Here's how the part is built. I have some questions about the finished solid (model axes, mm). A direction names the side the tool comes from. Round coordinates to 2 decimals unless told otherwise and drop trailing zeros. Write each loop counter-clockwise with the first axis right and the second up, starting at its lowest first coordinate (ties: lowest second). Pieces come first, ordered by that corner, then holes. Notation, with made-up numbers: (80, -29.75) - (121, -29.75) arc R21 ccw to (121, -12.75) - close; hole circle Ø10 at (42.25, 7). An arc over 180 degrees is marked (long way). Return JSON: item names as keys, results as strings. Group by question number.
```python
from build123d import *

# Parameters (mm, degrees)
SKETCH1_W                = 34.714871786
SKETCH1_H                = 6
BOSS_EXTRUDE1_DEPTH      = 1
BOSS_EXTRUDE2_DEPTH      = 11
BOSS_EXTRUDE3_DEPTH      = 5
BOSS_EXTRUDE3_DEPTH_BACK = 3
SKETCH3_W                = 50
SKETCH3_H                = 7
CUT_EXTRUDE3_DEPTH       = 25
SKETCH5_W                = 50
SKETCH5_H                = 7
CUT_EXTRUDE4_DEPTH       = 25
SKETCH6_W                = 50
SKETCH6_H                = 7
CUT_EXTRUDE5_DEPTH       = 25
SKETCH8_R                = 1.500000001
SKETCH8_R_2              = 1.499999999
BOSS_EXTRUDE5_DEPTH      = 1
BOSS_EXTRUDE10_DEPTH     = 3
REVOLVE1_ANGLE           = 90
SKETCH15_W               = 7.87412369
SKETCH15_H               = 12.308031651
CUT_EXTRUDE7_DEPTH       = 38


with BuildPart() as part:
    # Sketch1 → Boss-Extrude1 (new body)
    with BuildSketch(Plane(origin=(0, 0, 0), x_dir=(1, 0, 0), z_dir=(0, 1, 0))):
        Polygon((243.304219779, -116.484791863), (254.809280582, -136.408896135), (442.60209075, -136.409305398), (444.621046679, -132.925433226), (441.749040748, -132.925433226), (449.516726724, -119.47140646), (450.964695301, -121.978953126), (452.699916625, -118.984688022), (358.778179038, 43.666038061), (335.767496282, 43.666038061), align=None)
        with Locations((422.370878913, -131.984588005)):
            Rectangle(SKETCH1_W, SKETCH1_H, mode=Mode.SUBTRACT)
        Polygon((450.119365975, -117.364996826), (444.923425166, -120.365363323), (427.455346217, -90.114690822), (432.651287025, -87.114324326), align=None, mode=Mode.SUBTRACT)
        Polygon((428.11367092, -116.417164682), (266.43910827, -116.428009228), (347.273609731, 23.609230811), align=None, mode=Mode.SUBTRACT)
    extrude(amount=BOSS_EXTRUDE1_DEPTH)

    # Sketch1_9 → Boss-Extrude2 (add)
    # profile 1 of 2: a face of its own
    with BuildSketch(Plane(origin=(0, 0, 0), x_dir=(1, 0, 0), z_dir=(0, 1, 0))):
        Polygon((229.15943255, -134.984249185), (231.716666588, -139.412373829), (462.829865412, -139.412373829), (465.38624875, -134.984588004), (349.829542096, 65.165499075), (344.716133219, 65.165499075), align=None)
        Polygon((251.922647994, -136.409305396), (233.446303405, -136.408896135), (232.623553965, -134.984217354), (241.860901694, -118.984688016), align=None, mode=Mode.SUBTRACT)
        Polygon((442.60209075, -136.409305398), (254.809280582, -136.408896135), (243.304219779, -116.484791863), (335.767496282, 43.666038061), (358.778179038, 43.666038061), (461.938967961, -134.98458801), (461.116393749, -136.409305398), align=None, mode=Mode.SUBTRACT)
        Polygon((348.096628302, 62.164013367), (357.334800991, 46.166038067), (337.210874326, 46.166038067), (346.44844193, 62.165948237), align=None, mode=Mode.SUBTRACT)
    # profile 2 of 2: a face of its own
    with BuildSketch(Plane(origin=(0, 0, 0), x_dir=(1, 0, 0), z_dir=(0, 1, 0))):
        Polygon((441.749040748, -132.925433226), (444.621046679, -132.925433226), (450.964695301, -121.978953126), (449.516726724, -119.47140646), align=None)
    extrude(amount=BOSS_EXTRUDE2_DEPTH)

    # Sketch1_10 → Boss-Extrude3 (add, two sides: drawn at the far end of the back side and taken through both)
    # profile 1 of 2: a face of its own
    with BuildSketch(Plane(origin=(0, 0, 0), x_dir=(1, 0, 0), z_dir=(0, 1, 0)).offset(-BOSS_EXTRUDE3_DEPTH_BACK)):
        Polygon((229.15943255, -134.984249185), (231.716666588, -139.412373829), (462.829865412, -139.412373829), (465.38624875, -134.984588004), (349.829542096, 65.165499075), (344.716133219, 65.165499075), align=None)
        Polygon((251.922647994, -136.409305396), (233.446303405, -136.408896135), (232.623553965, -134.984217354), (241.860901694, -118.984688016), align=None, mode=Mode.SUBTRACT)
        Polygon((442.60209075, -136.409305398), (254.809280582, -136.408896135), (243.304219779, -116.484791863), (335.767496282, 43.666038061), (358.778179038, 43.666038061), (461.938967961, -134.98458801), (461.116393749, -136.409305398), align=None, mode=Mode.SUBTRACT)
        Polygon((348.096628302, 62.164013367), (357.334800991, 46.166038067), (337.210874326, 46.166038067), (346.44844193, 62.165948237), align=None, mode=Mode.SUBTRACT)
    # profile 2 of 2: a face of its own
    with BuildSketch(Plane(origin=(0, 0, 0), x_dir=(1, 0, 0), z_dir=(0, 1, 0)).offset(-BOSS_EXTRUDE3_DEPTH_BACK)):
        Polygon((441.749040748, -132.925433226), (444.621046679, -132.925433226), (450.964695301, -121.978953126), (449.516726724, -119.47140646), align=None)
    extrude(amount=BOSS_EXTRUDE3_DEPTH + BOSS_EXTRUDE3_DEPTH_BACK)

    # Sketch3 → Cut-Extrude3 (cut)
    with BuildSketch(Plane(origin=(290.589645397, 0, -167.772009994), x_dir=(-0.49999999999998745, 0, -0.8660254037844459), z_dir=(0.8660254037844459, 0, -0.49999999999998745))):
        with Locations((-236.592990632, -3)):
            Rectangle(SKETCH3_W, SKETCH3_H)
    extrude(amount=-CUT_EXTRUDE3_DEPTH, mode=Mode.SUBTRACT)

    # Sketch5 → Cut-Extrude4 (cut)
    with BuildSketch(Plane.XY.offset(139.412373829)):
        with Locations((347.273266, -3)):
            Rectangle(SKETCH5_W, SKETCH5_H)
    extrude(amount=-CUT_EXTRUDE4_DEPTH, mode=Mode.SUBTRACT)

    # Sketch6 → Cut-Extrude5 (cut)
    with BuildSketch(Plane(origin=(230.319375802, 0, 132.975171836), x_dir=(-0.5000006153901599, 0, 0.8660250484884727), z_dir=(-0.8660250484884727, 0, -0.5000006153901599))):
        with Locations((-113.236674797, -3)):
            Rectangle(SKETCH6_W, SKETCH6_H)
    extrude(amount=-CUT_EXTRUDE5_DEPTH, mode=Mode.SUBTRACT)

    # Sketch8 → Boss-Extrude5 (add)
    with BuildSketch(Plane.XZ.offset(3)):
        Polygon((349.829542096, -65.165499075), (465.38624875, 134.984588004), (462.829865412, 139.412373829), (231.716666588, 139.412373829), (229.15943255, 134.984249185), (344.716133219, -65.165499075), align=None)
        with Locations(Location((395.323540807, 98.692824233, 0), (0, 0, 270))):
            Circle(SKETCH8_R, mode=Mode.SUBTRACT)
        with Locations(Location((348.301285092, 15.86352663, 0), (0, 0, 270))):
            Circle(SKETCH8_R_2, mode=Mode.SUBTRACT)
        with Locations(Location((299.654911442, 97.241681778, 0), (0, 0, 270))):
            Circle(SKETCH8_R, mode=Mode.SUBTRACT)
        Polygon((444.621046678, 132.925433226), (450.9646953, 121.978953126), (449.516726723, 119.47140646), (427.347592194, 115.090208206), (404.332986149, 103.060878104), (405.774939108, 100.430142149), (424.549299543, 110.243170392), (451.871255231, 117.549638152), (452.699916625, 118.984688022), (461.93896796, 134.98458801), (461.116393748, 136.409305398), (442.602090749, 136.409305398), (439.019602541, 136.409297591), (420.379437569, 116.417683466), (402.410382204, 106.568526043), (403.852335163, 103.937790089), (426.620208945, 116.417264858), (441.749040748, 132.925433226), align=None, mode=Mode.SUBTRACT)
        Polygon((322.273266, 116.424264074), (294.35821863, 68.061097963), (319.354499369, 24.757680454), (376.473657314, 26.969372807), (401.472679509, 70.271207532), (372.273266, 116.420910254), align=None, mode=Mode.SUBTRACT)
        Polygon((233.446303405, 136.408896135), (251.922647993, 136.409305396), (241.860901693, 118.984688015), (232.623553964, 134.984217354), align=None, mode=Mode.SUBTRACT)
        Polygon((337.210874326, -46.166038067), (357.334800991, -46.166038067), (348.096628302, -62.164013367), (346.44844193, -62.165948237), align=None, mode=Mode.SUBTRACT)
    extrude(amount=BOSS_EXTRUDE5_DEPTH)

    # Sketch12 → Boss-Extrude10 (add)
    with BuildSketch(Plane(origin=(0, -3, 0), x_dir=(1, 0, 0), z_dir=(0, 1, 0))):
        with BuildLine():
            Line((347.417900212, -11.962292063), (347.307477102, -11.474637742))
            ThreePointArc((347.307477102, -11.474637741), (345.119304576, -12.681546115), (343.912396203, -14.86971864))
            Line((343.912396203, -14.86971864), (344.400050524, -14.98014175))
            ThreePointArc((344.400050524, -14.98014175), (345.472857967, -13.035099505), (347.417900212, -11.962292062))
        make_face()
        with BuildLine():
            ThreePointArc((352.690173981, -14.86971864), (351.483265607, -12.681546115), (349.295093082, -11.474637741))
            Line((349.295093082, -11.474637742), (349.184669972, -11.962292063))
            ThreePointArc((349.184669972, -11.962292062), (351.129712217, -13.035099505), (352.20251966, -14.98014175))
            Line((352.20251966, -14.98014175), (352.690173981, -14.86971864))
        make_face()
        with BuildLine():
            ThreePointArc((349.295093082, -20.25241552), (351.483265607, -19.045507146), (352.690173981, -16.85733462))
            Line((352.690173981, -16.85733462), (352.20251966, -16.74691151))
            ThreePointArc((352.20251966, -16.74691151), (351.129712217, -18.691953755), (349.184669972, -19.764761199))
            Line((349.184669972, -19.764761198), (349.295093082, -20.252415519))
        make_face()
        with BuildLine():
            Line((344.400050524, -16.74691151), (343.912396203, -16.85733462))
            ThreePointArc((343.912396203, -16.85733462), (345.119304576, -19.045507146), (347.307477102, -20.25241552))
            Line((347.307477102, -20.252415519), (347.417900212, -19.764761198))
            ThreePointArc((347.417900212, -19.764761199), (345.472857967, -18.691953755), (344.400050524, -16.74691151))
        make_face()
        with BuildLine():
            Line((394.440155927, -94.791589665), (394.329732817, -94.303935344))
            ThreePointArc((394.329732817, -94.303935343), (392.141560291, -95.510843717), (390.934651917, -97.699016243))
            Line((390.934651918, -97.699016243), (391.424789599, -97.798542944))
            ThreePointArc((391.424789599, -97.798542944), (392.499067688, -95.860448621), (394.440155927, -94.791589664))
        make_face()
        with BuildLine():
            ThreePointArc((399.712429696, -97.699016243), (398.505521322, -95.510843717), (396.317348797, -94.303935343))
            Line((396.317348797, -94.303935344), (396.206925687, -94.791589665))
            ThreePointArc((396.206925687, -94.791589664), (398.151967932, -95.864397108), (399.224775375, -97.809439353))
            Line((399.224775375, -97.809439353), (399.712429695, -97.699016243))
        make_face()
        with BuildLine():
            ThreePointArc((396.317348797, -103.081713122), (398.505521322, -101.874804748), (399.712429696, -99.686632223))
            Line((399.712429695, -99.686632223), (399.224775375, -99.576209113))
            ThreePointArc((399.224775375, -99.576209113), (398.151967932, -101.521251358), (396.206925687, -102.594058801))
            Line((396.206925687, -102.5940588), (396.317348797, -103.081713121))
        make_face()
        with BuildLine():
            Line((391.422306239, -99.576209113), (390.934651918, -99.686632223))
            ThreePointArc((390.934651917, -99.686632223), (392.141560291, -101.874804748), (394.329732817, -103.081713122))
            Line((394.329732817, -103.081713121), (394.440155927, -102.5940588))
            ThreePointArc((394.440155927, -102.594058801), (392.495113682, -101.521251358), (391.422306238, -99.576209113))
        make_face()
        with BuildLine():
            ThreePointArc((298.661103452, -92.85279289), (296.472930928, -94.059701263), (295.266022554, -96.247873788))
            Line((295.266022553, -96.247873788), (295.753676874, -96.358296898))
            ThreePointArc((295.753676875, -96.358296898), (296.826484318, -94.413254654), (298.771526562, -93.340447211))
            Line((298.771526562, -93.34044721), (298.661103452, -92.852792889))
        make_face()
        with BuildLine():
            ThreePointArc((304.04380033, -96.247873788), (302.836891957, -94.059701263), (300.648719432, -92.85279289))
            Line((300.648719432, -92.852792889), (300.538296322, -93.34044721))
            ThreePointArc((300.538296322, -93.340447211), (302.483338566, -94.413254654), (303.556146009, -96.358296898))
            Line((303.55614601, -96.358296898), (304.043800331, -96.247873788))
        make_face()
        with BuildLine():
            Line((300.538296322, -101.142916345), (300.648719432, -101.630570666))
            ThreePointArc((300.648719432, -101.630570665), (302.836891957, -100.423662292), (304.04380033, -98.235489767))
            Line((304.043800331, -98.235489768), (303.55614601, -98.125066658))
            ThreePointArc((303.556146009, -98.125066657), (302.483338566, -100.070108901), (300.538296322, -101.142916344))
        make_face()
        with BuildLine():
            Line((295.753676874, -98.125066658), (295.266022553, -98.235489768))
            ThreePointArc((295.266022554, -98.235489767), (296.472930928, -100.423662292), (298.661103452, -101.630570665))
            Line((298.661103452, -101.630570666), (298.771526562, -101.142916345))
            ThreePointArc((298.771526562, -101.142916344), (296.826484318, -100.070108901), (295.753676875, -98.125066657))
        make_face()
    extrude(amount=BOSS_EXTRUDE10_DEPTH)

    # Sketch13 → Revolve1 (revolve)
    with BuildSketch(Plane(origin=(0, 1, 0), x_dir=(1, 0, 0), z_dir=(0, 1, 0))):
        Polygon((448.425771751, -121.360995899), (428.11367092, -116.417164681), (442.800303922, -131.104591996), (443.050303922, -130.671579294), (428.985837114, -116.90637438), (448.175771751, -121.794008601), align=None)
    revolve(axis=Axis((442.800303922, 1, 131.104591996), (0.5000000000000009, 0, -0.8660254037844383)), revolution_arc=REVOLVE1_ANGLE)

    # Sketch15 → Cut-Extrude7 (cut)
    with BuildSketch(Plane(origin=(388.870181552, 0, 224.514303999), x_dir=(0.5000000000000009, -5.733535551193207e-15, -0.8660254037844383), z_dir=(0.8660254037844382, -9.930774881669059e-15, 0.5000000000000008))):
        with Locations((114.477088338, 17.154015826)):
            Rectangle(SKETCH15_W, SKETCH15_H)
    extrude(amount=-CUT_EXTRUDE7_DEPTH, mode=Mode.SUBTRACT)


solid = part.part
```
1) Imagine slicing it at B-B (y = 8). Give the number of separate pieces and of enclosed holes in the cut face, plus the area to 3 significant figures.
2) Will these pins go through, and if not, where does the flat tip stop? pin 1 Ø3.5 at (x, y) = (344, -1.5) entering from +Z; pin 2 Ø1 at (y, z) = (8, 25) entering from -X; pin 3 Ø1.8 at (x, z) = (351, 14) entering from +Y; pin 4 Ø4 at (x, y) = (374.5, 1) entering from -Z.
3) I need wall thicknesses on line 1 along Y through (x, z) = (366.5, -4); line 2 along Z through (x, y) = (246, 2.25); line 3 along Z through (x, y) = (431.5, 10.25). Which ranges of each line are inside material? Lowest first, please.
4) For faces 5 (the conical face through (441.948, 5.11, 120.563)), 6 (the flat face through (304.924, 0.168, 16.426)), 7 (the flat face through (387.128, 0.715, 45.424)), 8 (the flat face through (388.8, -3.49, 48.32)), which set-ups out of +Z, -Z, +X, -X, +Y, -Y let a thin tool reach every point of the face, with its end or its side?
5) If we mould it in two halves opening along Z, with no side actions, what happens to faces 1 (the flat face through (349, 4, 139.412)), 2 (the flat face through (408, 11, 37)), 3 (the conical face through (441.585, 5.484, 120.097)), 4 (the flat face through (406.8, 3.61, 33.51))? For each: released by +Z, released by -Z, zero draft, split by the parting line, or undercut.
6) Imagine slicing it at A-A (z = 64). Please give me the cut outline in (x, y).
7) Imagine slicing it at D-D (z = -20.5). Please give me the cut outline in (x, y), plus the area to 3 significant figures.
Results found:
{
 "1": {"separate pieces": "2", "enclosed holes": "4", "area": "2,250 mm²"},
 "2": {"pin 1": "stops at z = 139.41", "pin 2": "stops at x = 292.37", "pin 3": "stops at y = 0", "pin 4": "stops at z = -25.9"},
 "3": {"line 1": "y = -4 to -3, 0 to 1", "line 2": "z = 105.82 to 111.82, 121.15 to 126.15, 136.41 to 139.41", "line 3": "z = 76.29 to 82.27, 117.95 to 118.23, 118.51 to 118.89, 136.41 to 139.41"},
 "4": {"face 5": "none", "face 6": "-X", "face 7": "+Y", "face 8": "+Y, -Y"},
 "5": {"face 1": "released by +Z", "face 2": "zero draft", "face 3": "undercut", "face 4": "released by -Z"},
 "6": {"outline": "(270.14, -4) - (296.7, -4) - (296.7, -3) - (273.61, -3) - (273.61, 0) - (287.32, 0) - (287.32, 0.5) - (296.7, 0.5) - (296.7, 1) - (273.61, 1) - (273.61, 11) - (270.14, 11) - close; (397.85, -4) - (424.4, -4) - (424.4, 11) - (420.95, 11) - (420.95, 1) - (397.85, 1) - (397.85, 0.5) - (412.33, 0.5) - (412.33, 0) - (420.95, 0) - (420.95, -3) - (397.85, -3) - close"},
 "7": {"outline": "(318.93, -4) - (375.62, -4) - (375.62, 11) - (372.16, 11) - (372.16, 1) - (349.07, 1) - (349.07, 0) - (372.16, 0) - (372.16, -3) - (322.39, -3) - (322.39, 0) - (345.48, 0) - (345.48, 1) - (322.39, 1) - (322.39, 11) - (318.93, 11) - close", "area": "200 mm²"}
}
